Verification items for the finished model (mm, model axes). A direction names the side the tool comes from. Give positions to 0.01 mm unless a question says otherwise; leave off trailing zeros. Order: outer loops, then holes, each group sorted by start corner. A loop starts at its lowest first (then second) coordinate and runs counter-clockwise, first axis right, second up. Notation, with made-up numbers: (25, 16) - (75, 16) arc R27 ccw to (75, 42) - close; hole circle Ø3 at (6, 7). An arc over 180 degrees is marked (long way). Answer as a JSON object with one key per item and string values.
```python
from build123d import *

# Parameters (mm, degrees)
BOSS_EXTRUDE1_DEPTH = 50
SKETCH9_R           = 5
CUT_EXTRUDE1_DEPTH  = 87.602540378
SKETCH12_W          = 20
SKETCH12_H          = 15
CUT_EXTRUDE3_DEPTH  = 87.602540378


with BuildPart() as part:
    # Sketch1 → Boss-Extrude1 (new body)
    with BuildSketch(Plane.XY):
        Polygon((0, 0), (0, 15), (40, 50), (50, 50), (50, 0), align=None)
    extrude(amount=BOSS_EXTRUDE1_DEPTH)

    # Sketch9 → Cut-Extrude1 (cut, through all)
    with BuildSketch(Plane(origin=(0, 0, 0), x_dir=(-1, 0, 0), z_dir=(0, -1, 0))):
        with Locations(Location((-30, -25, 0), (0, 0, 90))):
            Circle(SKETCH9_R)
    extrude(amount=-CUT_EXTRUDE1_DEPTH, mode=Mode.SUBTRACT)

    # Sketch12 → Cut-Extrude3 (cut, through all)
    with BuildSketch(Plane(origin=(0, 0, 0), x_dir=(-1, 0, 0), z_dir=(0, -1, 0))):
        with Locations((-10, -25)):
            Rectangle(SKETCH12_W, SKETCH12_H)
    extrude(amount=-CUT_EXTRUDE3_DEPTH, mode=Mode.SUBTRACT)


solid = part.part
```
(1) Access from +Z, -Z, +X, -X, +Y, -Y to the whole of each face (thin tool, end or side, straight path). Record for faces 1 (the flat face through (10, 12, 17.5)), 2 (the flat face through (0, 7, 41)).
Computed values:
{"face 1": "-X, +Y, -Y", "face 2": "+Z, -Z, -X, +Y, -Y"}
(2) Release check for a two-part mould opening along X. For faces 3 (the cylindrical face through (34.957, 22.545, 25.651)), 4 (the flat face through (24, 36, 25)), 5 (the flat face through (10, 12, 32.5)), 6 (the flat face through (50, 25, 25)) record: pulls with the +X half, pulls with the -X half, needs draft (parallel to the pull), parting line crosses it, or undercut.
Computed values:
{"face 3": "undercut", "face 4": "pulls with the -X half", "face 5": "needs draft", "face 6": "pulls with the +X half"}
(3) Section check A-A (x = 30). Record the cut outline in (y, z).
Computed values:
{"outline": "(0, 0) - (41.25, 0) - (41.25, 20) - (0, 20) - close; (0, 30) - (41.25, 30) - (41.25, 50) - (0, 50) - close"}
(4) Section check B-B (z = 24). Record the cut outline in (x, y), then the cut area to 3 significant figures.
Computed values:
{"outline": "(20, 0) - (25.1, 0) - (25.1, 36.96) - (20, 32.5) - close; (34.9, 0) - (50, 0) - (50, 50) - (40, 50) - (34.9, 45.54) - close", "area": "921 mm²"}
(5) Section check D-D (x = 17). Record the cut outline in (y, z) (3 decimals), then the cut area to 3 significant figures.
Computed values:
{"outline": "(0, 0) - (29.875, 0) - (29.875, 17.5) - (0, 17.5) - close; (0, 32.5) - (29.875, 32.5) - (29.875, 50) - (0, 50) - close", "area": "1,050 mm²"}
(6) Section check C-C (y = 26). Record the cut outline in (x, z).
Computed values:
{"outline": "(12.57, 0) - (50, 0) - (50, 50) - (12.57, 50) - (12.57, 32.5) - (20, 32.5) - (20, 17.5) - (12.57, 17.5) - close; hole circle Ø10 at (30, 25)"}
(7) Gauge pin test, flat ends, axial feed: pin 1 Ø8 at (x, z) = (25, 45) entering from +Y (3 decimals); pin 2 Ø6 at (y, z) = (23, 32.5) entering from -X; pin 3 Ø10 at (x, y) = (35, 44) entering from -Z; pin 4 Ø6 at (x, z) = (24.5, 7.5) entering from +Y. Record the tip position at first contact, or that the pin passes through.
Computed values:
{"pin 1": "stops at y = 40.375", "pin 2": "stops at x = 5.71", "pin 3": "stops at z = 0", "pin 4": "stops at y = 39.06"}
(8) Material ranges on line 1 along X through (y, z) = (20.5, 25); line 2 along Z through (x, y) = (19, 30); line 3 along Z through (x, y) = (30, 15), recorded low to high. Write a range as [from, to].
Computed values:
{"line 1": "x = [20, 25], [35, 50]", "line 2": "z = [0, 17.5], [32.5, 50]", "line 3": "z = [0, 20], [30, 50]"}
